from build123d import *

# Parameters (mm, degrees)
SKETCH_1_R               = 11
SKETCH_1_R_2             = 5
EXTRUDE_1_DEPTH          = 2.2
SKETCH_2_R               = 5
EXTRUDE_2_DEPTH          = 10
F_3_0MM_1_D              = 3
PATTERN_CIRCULAR_1_COUNT = 4
CHAMFER_3_SIZE           = 0.2
SKETCH_12_R              = 2.5
EXTRUDE_1789_DEPTH       = 26
CUT_EXTRUDE_START        = -15
CUT_EXTRUDE_1_DEPTH      = 15


with BuildPart() as part:
    # 草图1 → 凸台-拉伸1 (new body)
    # profile 1 of 2: a face of its own
    with BuildSketch(Plane.XY):
        Circle(SKETCH_1_R)
        Circle(SKETCH_1_R_2, mode=Mode.SUBTRACT)
    # profile 2 of 2: a face of its own
    with BuildSketch(Plane.XY):
        Circle(SKETCH_1_R_2)
    extrude(amount=EXTRUDE_1_DEPTH)

    # 草图2 → 凸台-拉伸2 (add)
    with BuildSketch(Plane.XY.offset(2.2)):
        Circle(SKETCH_2_R)
    extrude(amount=EXTRUDE_2_DEPTH)

    # Ø3.0mm 暗销孔1 (through all)
    with Locations(Plane.XY.offset(2.2)):
        with Locations((0, 8)):
            f_3_0mm_1 = Hole(F_3_0MM_1_D / 2)

    # 阵列(圆周)1: Ø3.0mm 暗销孔1 ×4 about axis
    pattern_circular_1_axis = Axis((0, 0, 0), (0, 0, 1))
    for i in range(1, PATTERN_CIRCULAR_1_COUNT):
        add(f_3_0mm_1.rotate(pattern_circular_1_axis, i * 360 / PATTERN_CIRCULAR_1_COUNT), mode=Mode.SUBTRACT)

    # 倒角3
    chamfer_3_edges = [part.edges().sort_by_distance(p)[0] for p in [
        (-11, 0, 0),
        (-11, 0, 2.2),
    ]]
    chamfer(chamfer_3_edges, length=CHAMFER_3_SIZE)

    # 草图12 → Extrude 1789 (add)
    with BuildSketch(Plane.XY.offset(2.2)):
        with Locations(Location((0, 0, 0), (0, 0, 180))):
            Circle(SKETCH_12_R)
    extrude(amount=EXTRUDE_1789_DEPTH)

    # 草图13 → 切除-拉伸1 (cut)
    with BuildSketch(Plane.XY.offset(28.2).offset(CUT_EXTRUDE_START)):
        with BuildLine():
            Line((1.5, 2), (1.5, -2))
            ThreePointArc((1.5, -2), (2.5, 0), (1.5, 2))
        make_face()
    extrude(amount=CUT_EXTRUDE_1_DEPTH, mode=Mode.SUBTRACT)


solid = part.part
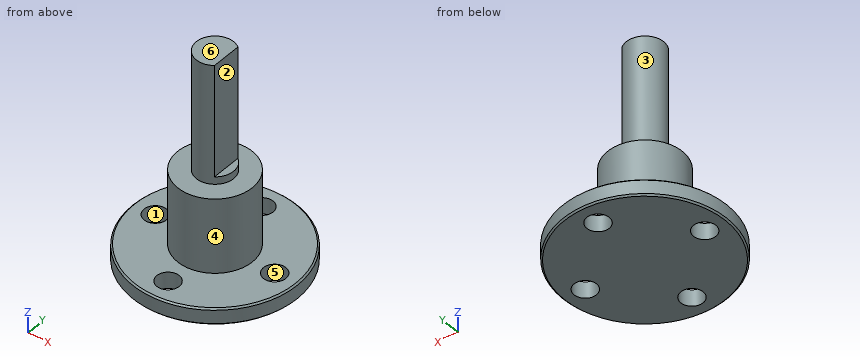
Read the model definition and answer for the solid it produces. Units are mm, in the model's axes. Face numbers are marked on the shaded views. A direction names the side the tool comes from. Round coordinates to 2 decimals unless told otherwise and drop trailing zeros. Write each loop counter-clockwise with the first axis right and the second up, starting at its lowest first coordinate (ties: lowest second). Pieces come first, ordered by that corner, then holes. Notation, with made-up numbers: (-39.5, -18.75) - (-23.5, -18.75) arc R23 cw to (-23.5, 11.25) - close; hole circle Ø6 at (-1, 0.25). An arc over 180 degrees is marked (long way). One line per question, with ' | ' between items. Start each with the question number.
1. For the marked faces 1, 2 and 3, determine the directions among +Z, -Z, +X, -X, +Y, -Y from which every point of the face is accessible in a straight line to the end or side of a thin tool.
2. Section A-A (y = 0) is taken. Determine the outline of the cut face in (x, z), and give its area (3 significant figures).
3. For a pull along X with two mould halves and no side action, classify the marked faces 4, 5 and 6 as +X half, -X half, draft (parallel to the pull), parting line (faces both ways), or undercut.
4. Section B-B (x = 0) is taken. Determine the outline of the cut face in (y, z), and give its area (3 significant figures).
5. Find the intervals of material crossed by probe 1 along Y at (x, z) = (0, 1.25); probe 2 along Z at (x, y) = (-3.75, 5.25); probe 3 along X at (y, z) = (-8, 1.3), in increasing order. Write a range as [from, to].
6. Each of these flat-tipped pins is pushed along its axis until it touches: pin 1 (10 mm diameter, centred on x = 1.5, y = -3, fed in from +Z); pin 2 (5 mm diameter, centred on x = 0, y = -8, fed in from +Z); pin 3 (10 mm diameter, centred on x = -4, z = 21.5, fed in from -Y); pin 4 (10 mm diameter, centred on x = 0, z = 20, fed in from +Y). Where does it stop, or does it pass through?
7. Section C-C (z = 3.25) is taken. Determine the outline of the cut face in (x, y), and give its area (3 significant figures).
Filled in:
1) face 1: +Z, -Z | face 2: +Z, +X, +Y, -Y | face 3: +Z
2) outline: (-11, 0.2) - (-10.8, 0) - (-9.5, 0) - (-9.5, 2.2) - (-10.8, 2.2) - (-11, 2) - close; (-6.5, 0) - (6.5, 0) - (6.5, 2.2) - (5, 2.2) - (5, 12.2) - (2.5, 12.2) - (2.5, 13.2) - (1.5, 13.2) - (1.5, 28.2) - (-2.5, 28.2) - (-2.5, 12.2) - (-5, 12.2) - (-5, 2.2) - (-6.5, 2.2) - close; (9.5, 0) - (10.8, 0) - (11, 0.2) - (11, 2) - (10.8, 2.2) - (9.5, 2.2) - close | area: 200 mm²
3) face 4: parting line | face 5: undercut | face 6: draft
4) outline: (-11, 0.2) - (-10.8, 0) - (-9.5, 0) - (-9.5, 2.2) - (-10.8, 2.2) - (-11, 2) - close; (-6.5, 0) - (6.5, 0) - (6.5, 2.2) - (5, 2.2) - (5, 12.2) - (2.5, 12.2) - (2.5, 28.2) - (-2.5, 28.2) - (-2.5, 12.2) - (-5, 12.2) - (-5, 2.2) - (-6.5, 2.2) - close; (9.5, 0) - (10.8, 0) - (11, 0.2) - (11, 2) - (10.8, 2.2) - (9.5, 2.2) - close | area: 215 mm²
5) probe 1: [-11, -9.5], [-6.5, 6.5], [9.5, 11] | probe 2: [0, 2.2] | probe 3: [-7.55, -1.5], [1.5, 7.55]
6) pin 1: z = 28.2 | pin 2: z = 2.2 | pin 3: y = -2.5 | pin 4: y = 2.5
7) outline: circle Ø10 at (0, 0) | area: 78.5 mm²
